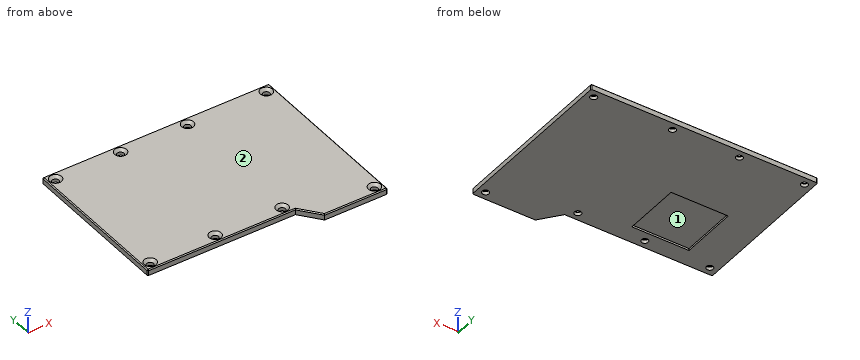
from build123d import *

# Parameters (mm, degrees)
PAD010_DEPTH        = 3
HOLE002_D           = 3.4
HOLE002_DEPTH       = 5
HOLE002_CSINK_D     = 6.1
HOLE002_CSINK_ANGLE = 90
SKETCH027_W         = 29
SKETCH027_H         = 29
POCKET009_DEPTH     = 1
CHAMFER001_SIZE     = 0.5


with BuildPart() as part:
    # Sketch022 (on Face1 of CopyPad011) → Pad010 (new body)
    with BuildSketch(Plane.XY.offset(24)):
        Polygon((-5, -7), (70, -7), (78, -17), (110, -17), (110, 71), (-5, 71), align=None)
    extrude(amount=PAD010_DEPTH)

    # Hole002
    with Locations(Plane.XY.offset(27)):
        with Locations((-1, 67), (106, 67), (106, -13), (-1, -3), (32, 67), (66, -3), (32, -3), (66, 67)):
            CounterSinkHole(HOLE002_D / 2, HOLE002_CSINK_D / 2, depth=HOLE002_DEPTH, counter_sink_angle=HOLE002_CSINK_ANGLE)

    # Sketch027 → Pocket009 (cut)
    with BuildSketch(Plane(origin=(0, 0, 24), x_dir=(1, 0, 0), z_dir=(0, 0, -1))):
        with Locations((27.5, -16.5)):
            Rectangle(SKETCH027_W, SKETCH027_H)
    extrude(amount=-POCKET009_DEPTH, mode=Mode.SUBTRACT)

    # Chamfer001
    chamfer001_edges = [part.edges().sort_by_distance(p)[0] for p in [
        (-5, 32, 27),
        (52.5, 71, 27),
        (110, 27, 27),
        (94, -17, 27),
        (74, -12, 27),
        (32.5, -7, 27),
        (110, 71, 25.5),
        (110, -17, 25.5),
        (-5, 71, 25.5),
        (-5, -7, 25.5),
    ]]
    chamfer(chamfer001_edges, length=CHAMFER001_SIZE)


with BuildPart() as part_1:
    # Body002 placement: moved
    add(part.part.moved(Location((0, 0, -2.5))))


solid = part_1.part
Could you check a few things on this model? Use its own coordinates, in mm. Face numbers are marked on the shaded views. A direction names the side the tool comes from. Give positions to 0.01 mm unless a question says otherwise; leave off trailing zeros. Order: outer loops, then holes, each group sorted by start corner. A loop starts at its lowest first (then second) coordinate and runs counter-clockwise, first axis right, second up.
Item 1: For the marked faces 1 and 2, which set-ups out of +Z, -Z, +X, -X, +Y, -Y let a thin tool reach every point of the face, with its end or its side?
Item 2: I'm going to push flat-ended pins straight in: pin 1 (4 mm diameter, centred on x = 106, y = 67, fed in from +Z); pin 2 (5.5 mm diameter, centred on x = -1, y = -3, fed in from +Z); pin 3 (4.5 mm diameter, centred on x = 106, y = -13, fed in from +Z); pin 4 (3 mm diameter, centred on x = -1, y = 67, fed in from +Z). Where does each tip first touch, or does it pass through?
Item 3: If we section it at D-D, the plane x = 66: Write out the boundary of the cut face in (y, z).
Item 4: I need wall thicknesses on line 1 (Y direction, x = 32, z = 21.8); line 2 (Y direction, x = -1, z = 22.7); line 3 (X direction, y = -3, z = 22.2). Which ranges of each line are inside material? Lowest first, please.
Item 5: If we section it at C-C, the plane y = -3: Write out the boundary of the cut face in (x, z).
Item 6: If we section it at A-A, the plane x = 32: Write out the boundary of the cut face in (y, z), plus the area to 3 significant figures.
Item 7: If we section it at B-B, the plane y = 67: Count the separate pieces of the cut face and the enclosed holes in it, plus the area to 3 significant figures.
Values:
1. face 1: -Z
1. face 2: +Z, +X, -X, +Y, -Y
2. pin 1: stops at z = 23.45
2. pin 2: stops at z = 24.2
2. pin 3: stops at z = 23.7
2. pin 4: passes through
3. outline: (-7, 21.5) - (-4.7, 21.5) - (-4.7, 23.15) - (-6.05, 24.5) - (-6.5, 24.5) - (-7, 24) - close; (-1.3, 21.5) - (65.3, 21.5) - (65.3, 23.15) - (63.95, 24.5) - (0.05, 24.5) - (-1.3, 23.15) - close; (68.7, 21.5) - (71, 21.5) - (71, 24) - (70.5, 24.5) - (70.05, 24.5) - (68.7, 23.15) - close
4. line 1: y = -7 to -4.7, -1.3 to 2, 31 to 65.3, 68.7 to 71
4. line 2: y = -7 to -4.7, -1.3 to 65.3, 68.7 to 71
4. line 3: x = -5 to -2.7, 0.7 to 30.3, 33.7 to 64.3, 67.7 to 110
5. outline: (-5, 21.5) - (-2.7, 21.5) - (-2.7, 23.15) - (-4.05, 24.5) - (-4.5, 24.5) - (-5, 24) - close; (0.7, 21.5) - (30.3, 21.5) - (30.3, 23.15) - (28.95, 24.5) - (2.05, 24.5) - (0.7, 23.15) - close; (33.7, 21.5) - (64.3, 21.5) - (64.3, 23.15) - (62.95, 24.5) - (35.05, 24.5) - (33.7, 23.15) - close; (67.7, 21.5) - (110, 21.5) - (110, 24) - (109.5, 24.5) - (69.05, 24.5) - (67.7, 23.15) - close
6. outline: (-7, 21.5) - (-4.7, 21.5) - (-4.7, 23.15) - (-6.05, 24.5) - (-6.5, 24.5) - (-7, 24) - close; (-1.3, 21.5) - (2, 21.5) - (2, 22.5) - (31, 22.5) - (31, 21.5) - (65.3, 21.5) - (65.3, 23.15) - (63.95, 24.5) - (0.05, 24.5) - (-1.3, 23.15) - close; (68.7, 21.5) - (71, 21.5) - (71, 24) - (70.5, 24.5) - (70.05, 24.5) - (68.7, 23.15) - close
6. area: 181 mm2
7. separate pieces: 5
7. enclosed holes: 0
7. area: 297 mm2
